The model under review builds one solid part; all positions refer to its coordinate system, in mm. Face numbers are marked on the shaded views. Round coordinates to 2 decimals unless told otherwise and drop trailing zeros. Order: outer loops, then holes, each group sorted by start corner. A loop starts at its lowest first (then second) coordinate and runs counter-clockwise, first axis right, second up. Notation, with made-up numbers: (60.5, 16.5) - (68.5, 16.5) arc R24 cw to (68.5, 28.5) - close; hole circle Ø11 at (79, 36). An arc over 180 degrees is marked (long way). One line per question, with ' | ' between items. Start each with the question number.
Item 1: Add section C-C on y = 50. State the section outline as (x, z) points, and give its area (3 significant figures).
Item 2: For L1, parallel to X at y = 48.5, z = -8; L2, parallel to Y at x = 7, z = -9; L3, parallel to Y at x = 8, z = -11.5, list the stretches that pass through material, from the lowest coordinate up. Write a range as [from, to].
Item 3: Add section D-D on z = -10.75. State the section outline as (x, y) points.
Item 4: Add section A-A on x = 27.5. State the section outline as (y, z) points.
Item 5: Draft analysis for pull direction X (two halves, no side actions). For the marked faces 1, 2, 3 and 4, state which applies: +X half, -X half, draft (parallel to the pull), parting line (faces both ways), or undercut.
Item 6: Insertion check: pin 1 Ø3 at (x, y) = (34.5, 15.5) entering from +Z. The pin has a flat end and moves straight along its axis. Give the tip position at first contact, or say it passes through.
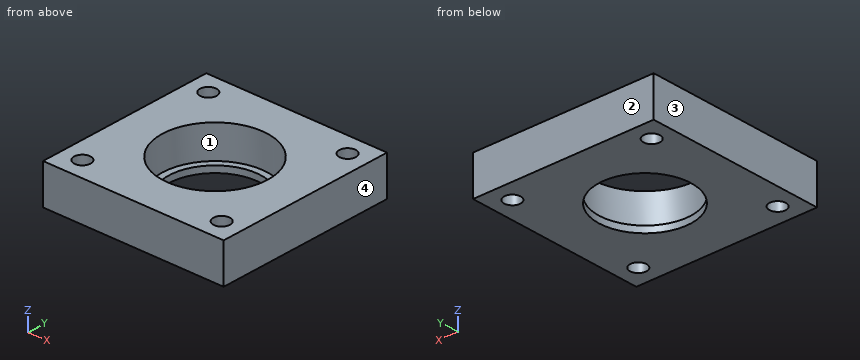
from build123d import *

# Parameters (mm, degrees)
SCHIZZO1_W                   = 55
SCHIZZO1_H                   = 55
ESTRUSIONE_ESTRUSIONE1_DEPTH = 12
SCHIZZO2_R                   = 16
TAGLIO_ESTRUSIONE1_DEPTH     = 10
SCHIZZO3_R                   = 14
TAGLIO_ESTRUSIONE2_DEPTH     = 10
SCHIZZO4_R                   = 2.5
TAGLIO_ESTRUSIONE3_DEPTH     = 79.70196948


with BuildPart() as part:
    # Schizzo1 → Estrusione-Estrusione1 (new body)
    with BuildSketch(Plane.XY):
        with Locations((27.5, 27.5)):
            Rectangle(SCHIZZO1_W, SCHIZZO1_H)
    extrude(amount=-ESTRUSIONE_ESTRUSIONE1_DEPTH)

    # Schizzo2 → Taglio-Estrusione1 (cut)
    with BuildSketch(Plane.XY):
        with Locations((27.5, 27.5)):
            Circle(SCHIZZO2_R)
    extrude(amount=-TAGLIO_ESTRUSIONE1_DEPTH, mode=Mode.SUBTRACT)

    # Schizzo3 → Taglio-Estrusione2 (cut)
    with BuildSketch(Plane.XY.offset(-10)):
        with Locations((27.5, 27.5)):
            Circle(SCHIZZO3_R)
    extrude(amount=-TAGLIO_ESTRUSIONE2_DEPTH, mode=Mode.SUBTRACT)

    # Schizzo4 → Taglio-Estrusione3 (cut, through all)
    with BuildSketch(Plane(origin=(0, 0, -12), x_dir=(-1, 0, 0), z_dir=(0, 0, -1))):
        with Locations((-48.713203436, 48.713203436)):
            Circle(SCHIZZO4_R)
        with Locations(Location((-6.286796564, 48.713203436, 0), (0, 0, 180))):
            Circle(SCHIZZO4_R)
        with Locations(Location((-48.713203436, 6.286796564, 0), (0, 0, 180))):
            Circle(SCHIZZO4_R)
        with Locations((-6.286796564, 6.286796564)):
            Circle(SCHIZZO4_R)
    extrude(amount=-TAGLIO_ESTRUSIONE3_DEPTH, mode=Mode.SUBTRACT)


solid = part.part
Determined:
1) outline: (0, -12) - (4.14, -12) - (4.14, 0) - (0, 0) - close; (8.43, -12) - (46.57, -12) - (46.57, 0) - (8.43, 0) - close; (50.86, -12) - (55, -12) - (55, 0) - (50.86, 0) - close | area: 557 mm2
2) L1: [0, 3.8], [8.78, 46.22], [51.2, 55] | L2: [0, 3.89], [8.68, 46.32], [51.11, 55] | L3: [0, 4.47], [8.11, 46.89], [50.53, 55]
3) outline: (0, 0) - (55, 0) - (55, 55) - (0, 55) - close; hole circle Ø5 at (6.29, 6.29); hole circle Ø5 at (6.29, 48.71); hole circle Ø28 at (27.5, 27.5); hole circle Ø5 at (48.71, 6.29); hole circle Ø5 at (48.71, 48.71)
4) outline: (0, -12) - (13.5, -12) - (13.5, -10) - (11.5, -10) - (11.5, 0) - (0, 0) - close; (41.5, -12) - (55, -12) - (55, 0) - (43.5, 0) - (43.5, -10) - (41.5, -10) - close
5) face 1: undercut | face 2: draft | face 3: -X half | face 4: +X half
6) pin 1: z = -10
